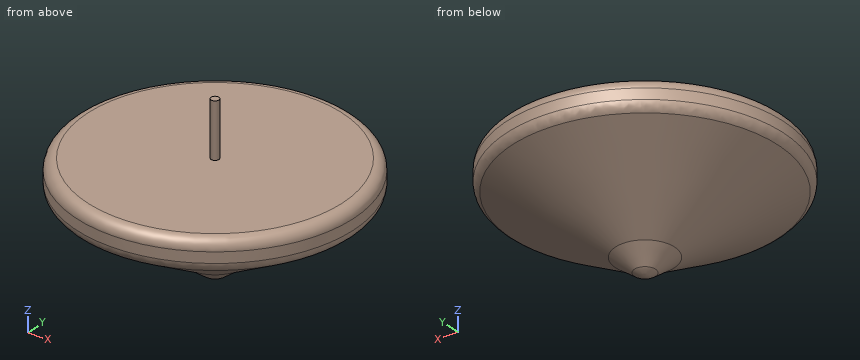
```python
from build123d import *

# Parameters (mm, degrees)
F2_R = 5.08


with BuildPart() as f1:
    # F0 (on Front) → F1 (revolve)
    with BuildSketch(Plane.XZ):
        with BuildLine():
            Line((4.890444, -6.616758), (13.825093, 0))
            Line((13.825093, 0), (64.812168, 29.610341))
            Line((64.812168, 29.610341), (64.812168, 42.566437))
            Line((64.812168, 42.566437), (1.862864, 42.566437))
            Line((1.862864, 42.566437), (1.862864, 68.062365))
            Line((1.862864, 68.062365), (0, 68.062365))
            Line((0, 68.062365), (0, -8.230456))
            ThreePointArc((0, -8.230456), (2.574901, -7.81661), (4.890444, -6.616758))
        make_face()
    revolve(axis=Axis((0, 0, 29.915955), (0, 0, -1)))

    # F2
    f2_edges = [f1.edges().sort_by_distance(p)[0] for p in [
        (-64.812168, 0, 42.566437),
        (-64.812168, 0, 29.610341),
    ]]
    fillet(f2_edges, radius=F2_R)


solid = f1.part
```
The model under review builds one solid part; all positions refer to its coordinate system, in mm. Round coordinates to 2 decimals unless told otherwise and drop trailing zeros. Write each loop counter-clockwise with the first axis right and the second up, starting at its lowest first coordinate (ties: lowest second). Pieces come first, ordered by that corner, then holes.
(1) Wall thickness on L1, parallel to Z at x = 51.5, y = -37; L2, parallel to Z at x = 3, y = -16.5; L3, parallel to Y at x = -54, z = 40: over which ranges is each line inside the solid? List them lowest first.
(2) We need section B-B on z = 14.5. Give the boundary of the cut face in (x, y), and give its area (3 significant figures).
(3) We need section A-A on z = 55. Give the boundary of the cut face in (x, y).
(4) Insertion check: pin 1 (1 mm diameter, centred on x = -27.5, y = -15.5, fed in from +Z); pin 2 (10 mm diameter, centred on y = 10.5, z = 42, fed in from -X); pin 3 (8 mm diameter, centred on y = 1.5, z = 38, fed in from -X); pin 4 (5 mm diameter, centred on x = -11, y = 50.5, fed in from -Z). Each pin has a flat end and moves straight along its axis. Give the tip position at first contact, or say it passes through.
Findings below:
1. L1: z = 29.03 to 40.99
1. L2: z = 1.71 to 42.57
1. L3: y = -34.62 to 34.62
2. outline: circle Ø77.59 at (0, 0)
2. area: 4,730 mm2
3. outline: circle Ø3.73 at (0, 0)
4. pin 1: stops at z = 42.57
4. pin 2: stops at x = -64.35
4. pin 3: stops at x = -64.81
4. pin 4: stops at z = 20.53
